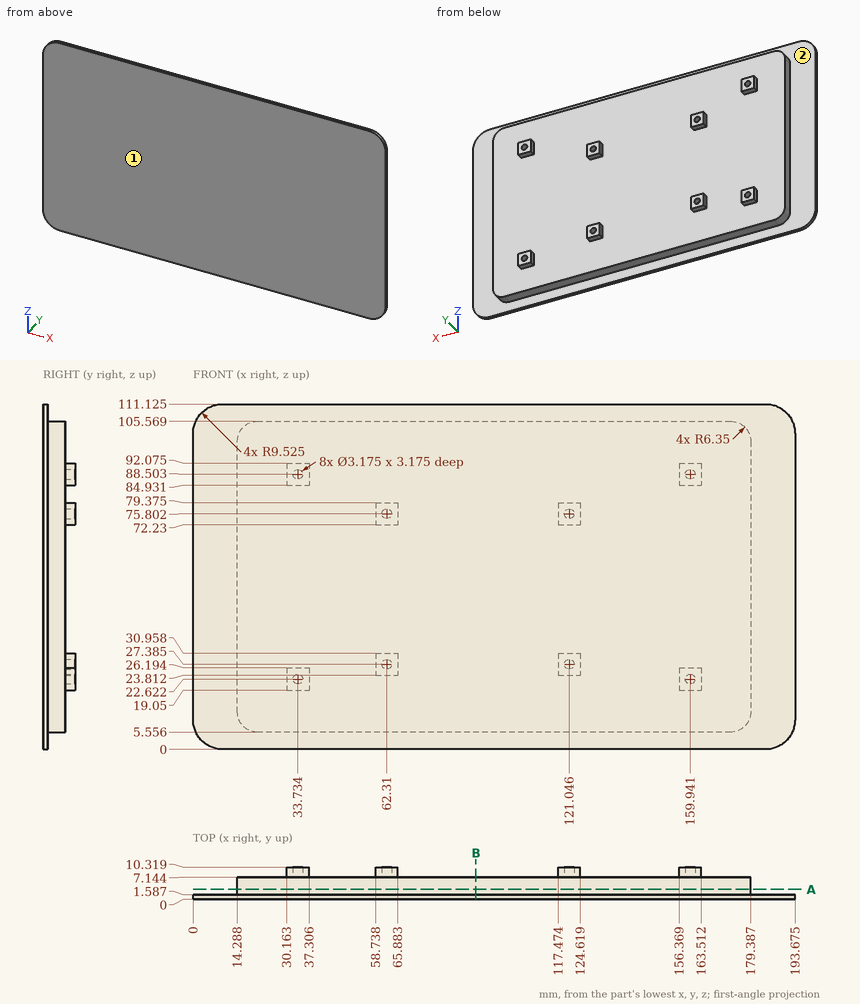
Input: dimensioned drawing with shaded views. Units: mm. Origin: part minimum x, y, z. A direction names the side the tool comes from. Coordinates: 2 decimals unless noted, no trailing zeros. Write each loop counter-clockwise with the first axis right and the second up, starting at its lowest first coordinate (ties: lowest second). Pieces come first, ordered by that corner, then holes. Notation, with made-up numbers: M 36.25,45.5 L 60.25,45.5 A16 cw 60.25,61.5 Z; hole C 9.25,46 d8. An arc over 180 degrees is marked long. Answer as a JSON object with one key per item and string values. Group by question number.
(1) Set-up query: the marked faces 1 and 2. Return all of +Z, -Z, +X, -X, +Y, -Y with unobstructed straight access to the full face (end or side cutting, diameter ignored); none if empty.
(2) Contact query for flat-ended pins moving along their axis: P1, Ø1, axis at y = 8.5, z = 88.5, coming from the -X side; P2, Ø3.5, axis at y = 8, z = 76, coming from the -X side; P3, Ø1.6, axis at x = 62.5, z = 76, coming from the +Y side. Output: stop coordinate, or through.
(3) Section B-B on x = 91. Output: boundary loops of the cut face in (y, z) (1 decimal), plus the area to 3 significant figures.
(4) Section A-A on y = 3.25. Output: boundary loops of the cut face in (x, z).
(5) Ray query, line 1 along X through (y, z) = (7.25, 78.5); line 2 along X through (y, z) = (6.5, 68); line 3 along X through (y, z) = (9, 87.5) (1 decimal). Return the intervals inside material, ascending. Write a range as [from, to].
Result set:
{
 "1": {"face 1": "+Z, -Z, +X, -X, -Y", "face 2": "+Y"},
 "2": {"P1": "stops at x = 30.16", "P2": "stops at x = 14.29", "P3": "stops at y = 7.14"},
 "3": {"outline": "M 0,0 L 1.6,0 L 1.6,5.6 L 7.1,5.6 L 7.1,105.6 L 1.6,105.6 L 1.6,111.1 L 0,111.1 Z", "area": "732 mm2"},
 "4": {"outline": "M 14.29,11.91 A6.35 ccw 20.64,5.56 L 173.04,5.56 A6.35 ccw 179.39,11.91 L 179.39,99.22 A6.35 ccw 173.04,105.57 L 20.64,105.57 A6.35 ccw 14.29,99.22 Z"},
 "5": {"line 1": "x = [58.74, 65.88], [117.47, 124.62]", "line 2": "x = [14.29, 179.39]", "line 3": "x = [30.2, 32.5], [35, 37.3], [156.4, 158.7], [161.2, 163.5]"}
}
